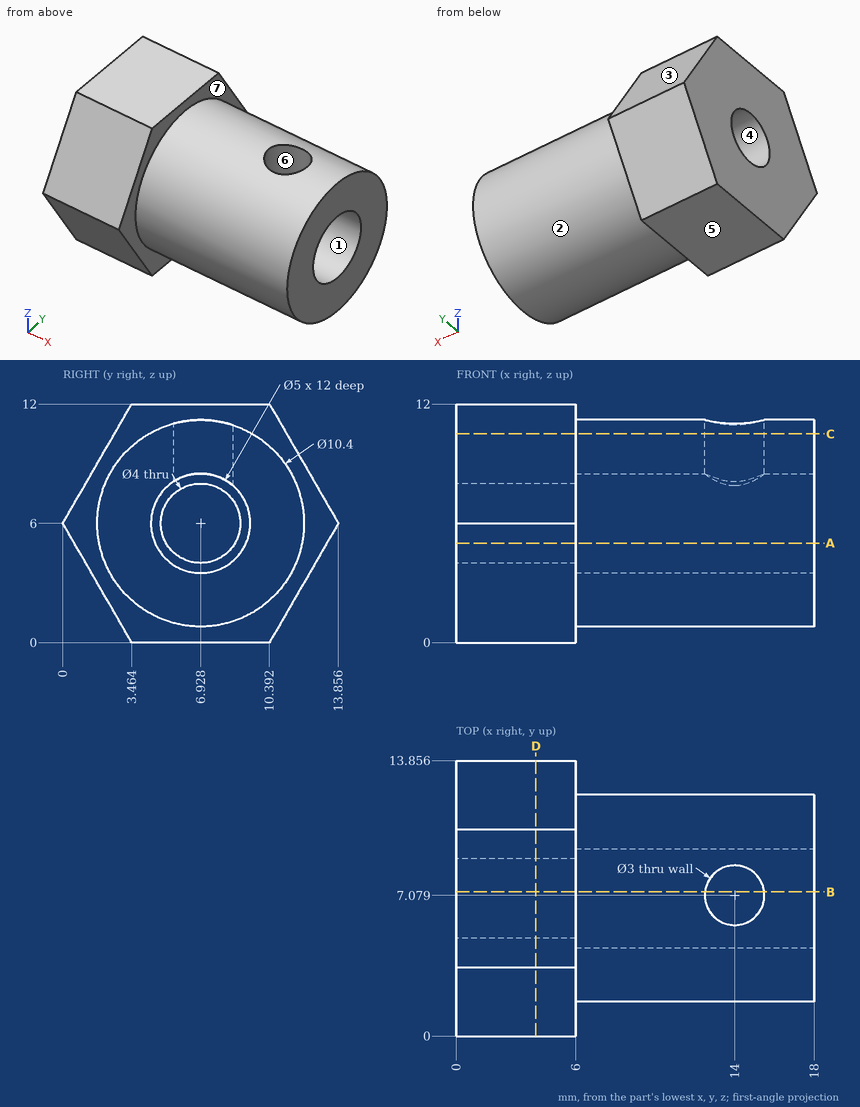
Study the drawing (mm; zero at the part's minimum x, y, z) and answer. A direction names the side the tool comes from. Give positions to 0.01 mm unless a question says otherwise; leave off trailing zeros. Loops run counter-clockwise (first coordinate to the right, second up) from the corner with the lowest first, then second, coordinate; pieces in that order, holes last. Notation, with made-up numbers: (16.5, 78) - (64.5, 78) arc R21 ccw to (64.5, 98) - close; hole circle Ø3 at (-21.75, 32.25). An arc over 180 degrees is marked (long way). Return JSON: item names as keys, results as strings. Group by question number.
1. Find section D-D (x = 4). Write down the section's boundary in (y, z).
2. Which of the six approach directions +Z, -Z, +X, -X, +Y, -Y give full straight-line access (tool end or side, diameter ignored) to the marked faces 5, 6 and 7?
3. Find section C-C (z = 10.5). Write down the section's boundary in (x, y).
4. Find section B-B (y = 7.25). Write down the section's boundary in (x, z), then the cut area to 3 significant figures.
5. Straight lines are drawn through the part: line 1 (X direction, y = 2.5, z = 10); line 2 (Z direction, x = 17.25, y = 7.5); line 3 (Z direction, x = 5.25, y = 6). For each, find the intervals that lie inside material, in ascending order. Write a range as [from, to].
6. Find section A-A (z = 5). Write down the section's boundary in (x, y) (1 decimal).
7. Determine the mould class of the marked faces 1, 2, 3 and 4 for opening direction Y: pulls with the +Y half, pulls with the -Y half, needs draft (parallel to the pull), parting line crosses it, or undercut.
8. Given pin 1 Ø5 at (x, z) = (3, 9.5) entering from +Y; pin 2 Ø1.5 at (x, y) = (13.5, 3) entering from +Z (1 decimal); pin 3 Ø4 at (x, y) = (14, 7.08) entering from -Z, each flat-ended and moving along its own axis, determine where each tip first touches the part or whether it passes through.
Verdict:
{
 "1": {"outline": "(0, 6) - (3.46, 0) - (10.39, 0) - (13.86, 6) - (10.39, 12) - (3.46, 12) - close; hole circle Ø4 at (6.93, 6)"},
 "2": {"face 5": "-Z, +X, -X, +Y, -Y", "face 6": "+Z", "face 7": "+X"},
 "3": {"outline": "(0, 2.6) - (6, 2.6) - (6, 4.32) - (18, 4.32) - (18, 9.53) - (6, 9.53) - (6, 11.26) - (0, 11.26) - close; hole circle Ø3 at (14, 7.08)"},
 "4": {"outline": "(0, 0) - (6, 0) - (6, 0.81) - (18, 0.81) - (18, 3.52) - (6, 3.52) - (6, 4.03) - (0, 4.03) - close; (0, 7.97) - (6, 7.97) - (6, 8.48) - (12.51, 8.48) - (12.51, 11.19) - (6, 11.19) - (6, 12) - (0, 12) - close; (15.49, 8.48) - (18, 8.48) - (18, 11.19) - (15.49, 11.19) - close", "area": "105 mm^2"},
 "5": {"line 1": "x = [0, 6]", "line 2": "z = [0.83, 3.57], [8.43, 11.17]", "line 3": "z = [0, 4.23], [7.77, 12]"},
 "6": {"outline": "(0, 0.6) - (6, 0.6) - (6, 1.8) - (18, 1.8) - (18, 4.6) - (6, 4.6) - (6, 5.2) - (0, 5.2) - close; (0, 8.7) - (6, 8.7) - (6, 9.2) - (18, 9.2) - (18, 12) - (6, 12) - (6, 13.3) - (0, 13.3) - close"},
 "7": {"face 1": "undercut", "face 2": "parting line crosses it", "face 3": "pulls with the +Y half", "face 4": "undercut"},
 "8": {"pin 1": "stops at y = 13.28", "pin 2": "stops at z = 10.1", "pin 3": "stops at z = 0.8"}
}
